```python
from build123d import *

# Parameters (mm, degrees)
SKETCH1_R           = 57
BOSS_EXTRUDE1_DEPTH = 25
SKETCH3_R           = 3
CUT_EXTRUDE1_DEPTH  = 104.556747728
CIRPATTERN1_COUNT   = 6


with BuildPart() as part:
    # Sketch1 → Boss-Extrude1 (new, symmetric)
    with BuildSketch(Plane.XY):
        with BuildLine():
            Line((6, 59.699246226), (6, 62))
            ThreePointArc((6, 62), (0, 68), (-6, 62))
            Line((-6, 62), (-6, 59.699246226))
            ThreePointArc((-6, 59.699246226), (-30, 51.961524227), (-48.701063819, 35.045775536))
            Line((-48.701063819, 35.045775536), (-50.693575035, 36.196152423))
            ThreePointArc((-50.693575035, 36.196152423), (-58.889727457, 34), (-56.693575035, 25.803847577))
            Line((-56.693575035, 25.803847577), (-54.701063819, 24.65347069))
            ThreePointArc((-54.701063819, 24.65347069), (-60, 0), (-54.701063819, -24.65347069))
            Line((-54.701063819, -24.65347069), (-56.693575035, -25.803847577))
            ThreePointArc((-56.693575035, -25.803847577), (-58.889727457, -34), (-50.693575035, -36.196152423))
            Line((-50.693575035, -36.196152423), (-48.701063819, -35.045775536))
            ThreePointArc((-48.701063819, -35.045775536), (-30, -51.961524227), (-6, -59.699246226))
            Line((-6, -59.699246226), (-6, -62))
            ThreePointArc((-6, -62), (0, -68), (6, -62))
            Line((6, -62), (6, -59.699246226))
            ThreePointArc((6, -59.699246226), (30, -51.961524227), (48.701063819, -35.045775536))
            Line((48.701063819, -35.045775536), (50.693575035, -36.196152423))
            ThreePointArc((50.693575035, -36.196152423), (58.889727457, -34), (56.693575035, -25.803847577))
            Line((56.693575035, -25.803847577), (54.701063819, -24.65347069))
            ThreePointArc((54.701063819, -24.65347069), (60, 0), (54.701063819, 24.65347069))
            Line((54.701063819, 24.65347069), (56.693575035, 25.803847577))
            ThreePointArc((56.693575035, 25.803847577), (58.889727457, 34), (50.693575035, 36.196152423))
            Line((50.693575035, 36.196152423), (48.701063819, 35.045775536))
            ThreePointArc((48.701063819, 35.045775536), (30, 51.961524227), (6, 59.699246226))
        make_face()
        Circle(SKETCH1_R, mode=Mode.SUBTRACT)
    extrude(amount=BOSS_EXTRUDE1_DEPTH, both=True)

    # Sketch3 → Cut-Extrude1 (cut, through all)
    with BuildSketch(Plane(origin=(0, 0, -25), x_dir=(-1, 0, 0), z_dir=(0, 0, -1))):
        with Locations((0, 62)):
            Circle(SKETCH3_R)
    cut_extrude1 = extrude(amount=-CUT_EXTRUDE1_DEPTH, mode=Mode.SUBTRACT)

    # CirPattern1: Cut-Extrude1 ×6 about axis
    cirpattern1_axis = Axis((0, 0, 0), (0, 0, 1))
    for i in range(1, CIRPATTERN1_COUNT):
        add(cut_extrude1.rotate(cirpattern1_axis, i * 360 / CIRPATTERN1_COUNT), mode=Mode.SUBTRACT)


solid = part.part
```
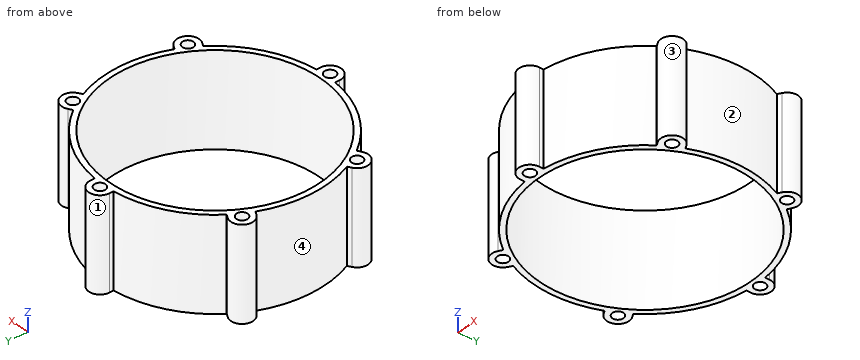
The listing builds one solid part. Answer for the finished solid, in the listing's coordinates (mm). Face numbers are marked on the shaded views. Coordinates: 2 decimals unless noted, no trailing zeros. Loops run counter-clockwise (first coordinate to the right, second up) from the corner with the lowest first, then second, coordinate; pieces in that order, holes last. Notation, with made-up numbers: (16, -35.5) - (51, -35.5) arc R17 cw to (51, -15.5) - close; hole circle Ø8 at (61.25, 50). An arc over 180 degrees is marked (long way). Use a Markdown table: item, result. Add a question column.
1) Find the intervals of material crossed by line 1 (Y direction, x = 0, z = 1); line 2 (X direction, y = 6, z = 22); line 3 (X direction, y = 31.5, z = -14), in increasing order.
2) The part is cut by section C-C, the plane z = -3. State how many separate pieces and enclosed holes the cut face has, and give its area (3 significant figures).
3) The mould has two halves that part along X. Classify the marked faces 1, 2, 3 and 4: released by +X, released by -X, zero draft, split by the parting line, or undercut.
4) The part is cut by section B-B, the plane x = 36.5. Give the vertices of the cut face in (y, z).
5) Given pin 1 (9.5 mm diameter, centred on x = -53.69, y = 31, fed in from +Z); pin 2 (0.7 mm diameter, centred on y = 60.5, z = 5.5, fed in from +X); pin 3 (6 mm diameter, centred on x = 29.5, z = -3, fed in from +Y); pin 4 (3 mm diameter, centred on y = 40, z = -8.5, fed in from +X), each flat-ended and moving along its own axis, determine where each tip first touches the part or whether it passes through.
6) The part is cut by section A-A, the plane y = 0. Give the vertices of the cut face in (x, z), and give its area (3 significant figures).
Here are the results:
| question | item | result |
|---|---|---|
| 1 | line 1 | y = -68 to -65, -59 to -57, 57 to 59, 65 to 68 |
| 1 | line 2 | x = -59.7 to -56.68, 56.68 to 59.7 |
| 1 | line 3 | x = -59.67 to -56.65, -50.74 to -47.51, 47.51 to 50.74, 56.65 to 59.67 |
| 2 | separate pieces | 1 |
| 2 | enclosed holes | 7 |
| 2 | area | 1,420 mm^2 |
| 3 | face 1 | split by the parting line |
| 3 | face 2 | released by +X |
| 3 | face 3 | undercut |
| 3 | face 4 | released by -X |
| 4 | outline | (-47.62, -25) - (-43.78, -25) - (-43.78, 25) - (-47.62, 25) - close; (43.78, -25) - (47.62, -25) - (47.62, 25) - (43.78, 25) - close |
| 5 | pin 1 | stops at z = 25 |
| 5 | pin 2 | stops at x = 6 |
| 5 | pin 3 | stops at y = 53.83 |
| 5 | pin 4 | stops at x = 46.02 |
| 6 | outline | (-60, -25) - (-57, -25) - (-57, 25) - (-60, 25) - close; (57, -25) - (60, -25) - (60, 25) - (57, 25) - close |
| 6 | area | 300 mm^2 |
